Work out the finished part from the listing and answer in its coordinate system (mm). A direction names the side the tool comes from. Coordinates: 2 decimals unless noted, no trailing zeros. Write each loop counter-clockwise with the first axis right and the second up, starting at its lowest first coordinate (ties: lowest second). Pieces come first, ordered by that corner, then holes. Notation, with made-up numbers: (69.25, -14) - (77.25, -14) arc R33 ccw to (77.25, 20) - close; hole circle Ø6 at (78, 20). An arc over 180 degrees is marked (long way). Use a Markdown table: item, result. Add a question column.
(1) Find the intervals of material crossed by line 1 (Y direction, x = 0, z = -4.45); line 2 (Y direction, x = 0, z = 1.35); line 3 (Y direction, x = 0, z = -0.85), in increasing order. Write a range as from..to.
(2) The part is cut by section A-A, the plane y = 0. Give the vertices of the cut face in (x, z), then the cut area to 3 significant figures.
(3) For a pull along Y with two mould halves and no side action, classify faces 4 (the face through (1.725, -13.137, 0.71)), 5 (the face through (-5, -5, -4.36)), 6 (the face through (2, -6, 1.44)) as released by +Y, released by -Y, zero draft, split by the parting line, or undercut.
(4) A tool of negligible diameter and unlimited length cuts with its end or side. For faces 1 (the face through (12, -2, 0)), 2 (the face through (-4, 11, 1.44)), 3 (the face through (-5, -5, 1.24)), from which of +Z, -Z, +X, -X, +Y, -Y can it reach the whole face along a straight path? Write none if from no direction.
(5) Given pin 1 Ø1.5 at (x, z) = (0, -3) entering from +Y; pin 2 Ø11 at (x, y) = (0, 0) entering from -Z; pin 3 Ø2 at (y, z) = (10, -3) entering from -X, each flat-ended and moving along its own axis, determine where each tip first touches the part or whether it passes through.
(6) The part is cut by section C-C, the plane x = 9.5. Give the vertices of the cut face in (y, z), then the cut area to 3 significant figures.
(7) The part is cut by section D-D, the plane y = -11. Give the vertices of the cut face in (x, z).
from build123d import *

# Parameters (mm, degrees)
SKETCH_1_R          = 13.25
SKETCH_1_R_2        = 12
EXTRUDE_1_DEPTH     = 1.44
EXTRUDE_START       = -6
SKETCH_2_R          = 12
SKETCH_2_R_2        = 6
EXTRUDE_2_DEPTH     = 6
SKETCH_3_R          = 11.5
SKETCH_3_R_2        = 6.5
CUT_EXTRUDE_1_DEPTH = 0.2


with BuildPart() as part:
    # 草图1 → 凸台-拉伸1 (new body)
    with BuildSketch(Plane.XY):
        with Locations(Location((0, 0, 0), (0, 0, 180))):
            Circle(SKETCH_1_R)
        with Locations(Location((0, 0, 0), (0, 0, 180))):
            Circle(SKETCH_1_R_2, mode=Mode.SUBTRACT)
    extrude(amount=EXTRUDE_1_DEPTH)

    # 草图2 → 凸台-拉伸2 (add)
    with BuildSketch(Plane.XY.offset(1.44).offset(EXTRUDE_START)):
        Circle(SKETCH_2_R)
        Circle(SKETCH_2_R_2, mode=Mode.SUBTRACT)
    extrude(amount=EXTRUDE_2_DEPTH)

    # 草图3 → 切除-拉伸1 (cut)
    with BuildSketch(Plane(origin=(0, 0, -4.56), x_dir=(-1, 0, 0), z_dir=(0, 0, -1))):
        Circle(SKETCH_3_R)
        Circle(SKETCH_3_R_2, mode=Mode.SUBTRACT)
    cut_extrude_1 = extrude(amount=-CUT_EXTRUDE_1_DEPTH, mode=Mode.SUBTRACT)

    # 镜向1: 切除-拉伸1 across plane
    add(cut_extrude_1.mirror(Plane(origin=(0, 0, -1.56), x_dir=(1, 0, 0), z_dir=(0, 0, -1))), mode=Mode.SUBTRACT)


solid = part.part
Model answer:
| question | item | result |
|---|---|---|
| 1 | line 1 | -12..-11.5, -6.5..-6, 6..6.5, 11.5..12 |
| 1 | line 2 | -13.25..-11.5, -6.5..-6, 6..6.5, 11.5..13.25 |
| 1 | line 3 | -12..-6, 6..12 |
| 2 | outline | (-13.25, 0) - (-12, 0) - (-12, -4.56) - (-11.5, -4.56) - (-11.5, -4.36) - (-6.5, -4.36) - (-6.5, -4.56) - (-6, -4.56) - (-6, 1.44) - (-6.5, 1.44) - (-6.5, 1.24) - (-11.5, 1.24) - (-11.5, 1.44) - (-13.25, 1.44) - close; (6, -4.56) - (6.5, -4.56) - (6.5, -4.36) - (11.5, -4.36) - (11.5, -4.56) - (12, -4.56) - (12, 0) - (13.25, 0) - (13.25, 1.44) - (11.5, 1.44) - (11.5, 1.24) - (6.5, 1.24) - (6.5, 1.44) - (6, 1.44) - close |
| 2 | area | 71.6 mm^2 |
| 3 | face 4 | split by the parting line |
| 3 | face 5 | undercut |
| 3 | face 6 | zero draft |
| 4 | face 1 | -Z |
| 4 | face 2 | +Z, +X, -X, +Y, -Y |
| 4 | face 3 | +Z |
| 5 | pin 1 | y = 12 |
| 5 | pin 2 | through |
| 5 | pin 3 | x = -7.94 |
| 6 | outline | (-9.24, 0) - (-7.33, 0) - (-7.33, -4.56) - (-6.48, -4.56) - (-6.48, -4.36) - (6.48, -4.36) - (6.48, -4.56) - (7.33, -4.56) - (7.33, 0) - (9.24, 0) - (9.24, 1.44) - (6.48, 1.44) - (6.48, 1.24) - (-6.48, 1.24) - (-6.48, 1.44) - (-9.24, 1.44) - close |
| 6 | area | 88.3 mm^2 |
| 7 | outline | (-7.39, 0) - (-4.8, 0) - (-4.8, -4.56) - (-3.35, -4.56) - (-3.35, -4.36) - (3.35, -4.36) - (3.35, -4.56) - (4.8, -4.56) - (4.8, 0) - (7.39, 0) - (7.39, 1.44) - (3.35, 1.44) - (3.35, 1.24) - (-3.35, 1.24) - (-3.35, 1.44) - (-7.39, 1.44) - close |
